For this review, take the finished solid that the model builds, in its own axes (mm). Face numbers are marked on the shaded views. A direction names the side the tool comes from. Round coordinates to 2 decimals unless told otherwise and drop trailing zeros. Order: outer loops, then holes, each group sorted by start corner. A loop starts at its lowest first (then second) coordinate and runs counter-clockwise, first axis right, second up.
Autodesk Inventor part; units mm, degrees
ref_plane "YZ Plane" through (0, 0, 0) normal (1, 0, 0) x (0, 1, 0)
ref_plane "XZ Plane" through (0, 0, 0) normal (0, 1, 0) x (-1, 0, 0)
ref_plane "XY Plane" through (0, 0, 0) normal (0, 0, 1) x (1, 0, 0)
sketch "Sketch1" plane through (0, 0, 0) normal (0, 1, 0) x (-1, 0, 0)
  line L0 (0, 0) -> (-30, 0)
  line L1 (-30, 0) -> (-30, -48)
  line L2 (-30, -48) -> (0, -48)
  line L3 (0, -48) -> (0, 0)
  circle A0 centre (-15, -24) radius 6.25
  circle A1 centre (-23.5, -32.5) radius 1.6
  circle A2 centre (-6.5, -32.5) radius 1.6
  circle A3 centre (-4.5, -44) radius 1.6
  circle A4 centre (-25.5, -44) radius 1.6
  circle A5 centre (-23.5, -15.5) radius 1.6
  circle A6 centre (-6.5, -15.5) radius 1.6
  circle A7 centre (-4.5, -4) radius 1.6
  circle A8 centre (-25.5, -4) radius 1.6
  line L4 (-4.5, -44) -> (-25.5, -44) construction
  line L5 (-25.5, -44) -> (-25.5, -4) construction
  line L6 (-6.5, -32.5) -> (-23.5, -32.5) construction
  line L7 (-23.5, -32.5) -> (-23.5, -15.5) construction
  point P0 (0, -24)
  point P1 (-15, -48)
  point P2 (-23.5, -24)
  point P3 (-30, -24)
  point P4 (-25.5, -24)
  point P5 (-15, -32.5)
  point P6 (-15, -44)
  dimension "d0" = 30
  dimension "d1" = 48
  dimension "d2" = 12.5
  dimension "d3" = 3.2
  dimension "d4" = 17
  dimension "d5" = 17
  dimension "d6" = 40
  dimension "d7" = 21
extrude "Extrusion1" add sketch "Sketch1" along normal blind 2
sketch "Sketch2" plane through (0, 0, 0) normal (0, 0, 1) x (1, 0, 0)
  line L0 (0, 0) -> (30, 0) construction
  line L1 (0, 0) -> (0, 24.5)
  line L2 (30, 0) -> (30, 24.5)
  arc A0 (8.75, 22.5) -> (21.25, 22.5) centre (15, 22.5) ccw
  line L3 (21.25, 22.5) -> (21.25, 24.5)
  line L4 (23.25, 26.5) -> (28, 26.5)
  line L5 (8.75, 22.5) -> (8.75, 24.5)
  line L6 (6.75, 26.5) -> (2, 26.5)
  arc A1 (8.75, 24.5) -> (6.75, 26.5) centre (6.75, 24.5) ccw
  arc A2 (2, 26.5) -> (0, 24.5) centre (2, 24.5) ccw
  arc A3 (30, 24.5) -> (28, 26.5) centre (28, 24.5) ccw
  arc A4 (23.25, 26.5) -> (21.25, 24.5) centre (23.25, 24.5) ccw
  circle A5 centre (27, 22.5) radius 1.4
  circle A6 centre (27, 10.5) radius 1.4
  circle A7 centre (15, 10.5) radius 1.4
  circle A8 centre (3, 10.5) radius 1.4
  circle A9 centre (3, 22.5) radius 1.4
  line L7 (3, 10.5) -> (27, 10.5) construction
  line L8 (0, 0) -> (30, 0)
  point P0 (0, 26.5)
  point P1 (30, 26.5)
  point P2 (15, 0)
  point P3 (15, 0)
  point P4 (15, 0)
  dimension "d10" = 26.5
  dimension "d11" = 26.5
  dimension "d12" = 12.5
  dimension "d13" = 22.5
  dimension "d14" = 2
  dimension "d15" = 2.8
  dimension "d16" = 12
  dimension "d17" = 24
extrude "Extrusion2" add sketch "Sketch2" along normal blind 2
fillet "Fillet1" radius 2 1 edges at (15, 0, 2)
ref_plane "Work Plane1" through (0, 0, -24) normal (0, 0, -1) x (-1, 0, 0)
sketch "Sketch3" plane through (0, 0, -24) normal (0, 0, -1) x (-1, 0, 0)
  point P0 (0, 0)
mirror "Mirror1" about plane through (0, 0, -24) normal (0, 0, -1) of "Extrusion2", "Fillet1"
properties part number "SmallerBracket"
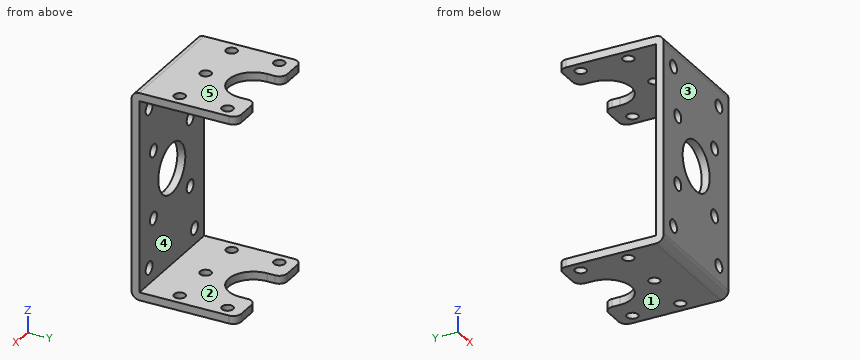
Q1. Wall thickness on line 1 (Z direction, x = 19.5, y = 9); line 2 (Y direction, x = 3, z = -48.35); line 3 (Y direction, x = 27, z = -49.05): over which ranges is each line inside the solid? List them lowest first.
Q2. Take a section at A-A, the plane z = -15.5. State the section outline as (x, y) points, plus the area to 3 significant figures.
Q3. Take a section at B-B, the plane x = 15. State the section outline as (y, z) points.
Q4. Take a section at D-D, the plane x = 22.5. State the section outline as (y, z) points, plus the area to 3 significant figures.
Q5. Tool access review of the marked faces 1 and 2: name each direction out of +Z, -Z, +X, -X, +Y, -Y from which nothing blocks a thin tool from reaching the whole face with its end or side.
Q6. Mouldability with a two-part tool opening along Z and no side actions: class the marked faces 3, 4 and 5 as +Z half, -Z half, draft (parallel to the pull), parting line (faces both ways), or undercut.
Q7. Take a section at C-C, the plane y = 3.5. State the section outline as (x, z) points, plus the area to 3 significant figures.
Q8. Clearance check with flat-ended pins moving along their axes: pin 1 (8 mm diameter, centred on x = 23.5, z = -16.5, fed in from -Y); pin 2 (3.5 mm diameter, centred on x = 25.5, z = -44, fed in from +Y). State where each tip first meets the part, or that it passes through.
Working result:
1. line 1: z = -50 to -48, 0 to 2
1. line 2: y = 0.03 to 9.1, 11.9 to 21.1, 23.9 to 26.5
1. line 3: y = 0.3 to 9.1, 11.9 to 21.1, 23.9 to 26.5
2. outline: (0, 0) - (4.9, 0) - (4.9, 2) - (0, 2) - close; (8.1, 0) - (21.9, 0) - (21.9, 2) - (8.1, 2) - close; (25.1, 0) - (30, 0) - (30, 2) - (25.1, 2) - close
2. area: 47.2 mm2
3. outline: (0, -48) arc R2 ccw to (2, -50) - (9.1, -50) - (9.1, -48) - (2, -48) - (2, -30.25) - (0, -30.25) - close; (0, -17.75) - (2, -17.75) - (2, 0) - (9.1, 0) - (9.1, 2) - (2, 2) arc R2 ccw to (0, 0) - close; (11.9, -50) - (16.25, -50) - (16.25, -48) - (11.9, -48) - close; (11.9, 0) - (16.25, 0) - (16.25, 2) - (11.9, 2) - close
4. outline: (0, -48) arc R2 ccw to (2, -50) - (26.35, -50) - (26.35, -48) - (2, -48) - (2, -33.75) - (0, -33.75) - close; (0, -31.25) - (2, -31.25) - (2, -16.75) - (0, -16.75) - close; (0, -14.25) - (2, -14.25) - (2, 0) - (26.35, 0) - (26.35, 2) - (2, 2) arc R2 ccw to (0, 0) - close
4. area: 190 mm2
5. face 1: -Z, +X, -X, +Y, -Y
5. face 2: +X, -X, +Y
6. face 3: draft
6. face 4: undercut
6. face 5: +Z half
7. outline: (0, -50) - (30, -50) - (30, -48) - (0, -48) - close; (0, 0) - (30, 0) - (30, 2) - (0, 2) - close
7. area: 120 mm2
8. pin 1: stops at y = 0
8. pin 2: stops at y = 2
